The drawing under review shows one solid part. Ordinate dimensions are in mm from its lowest x, y, z. A direction names the side the tool comes from. Coordinates: 2 decimals unless noted, no trailing zeros. Write each loop counter-clockwise with the first axis right and the second up, starting at its lowest first coordinate (ties: lowest second). Pieces come first, ordered by that corner, then holes.
Q1. Add section B-B, the plane y = 18. Give the boundary of the cut face in (x, z), plus the area to 4 significant figures.
Q2. Clearance check with flat-ended pins moving along their axes: pin 1 Ø7 at (y, z) = (20, 115) entering from +X; pin 2 Ø13.5 at (y, z) = (20, 35) entering from +X; pin 3 Ø4 at (x, z) = (38, 134) entering from +Y. State where each tip first meets the part, or that it passes through.
Q3. Add section D-D, the plane z = 57.5. Give the boundary of the cut face in (x, y).
Q4. Machinability: for the marked faces 1 and 2, which of the approach directions +Z, -Z, +X, -X, +Y, -Y give a long, thin tool a straight path to every point of the face, cutting with its end or side? Answer none if there is none.
Q5. To check wall thickness, follow probe 1 along Z at (x, y) = (6.75, 20); probe 2 along Y at (x, z) = (7.75, 75); probe 3 along X at (y, z) = (5.25, 125). State the ranges of each line that lie inside material, in increasing order.
Q6. Add section C-C, the plane z = 113. Give the boundary of the cut face in (x, y), plus the area to 4 significant figures.
Q7. Add section A-A, the plane z = 75. Give the boundary of the cut face in (x, y).
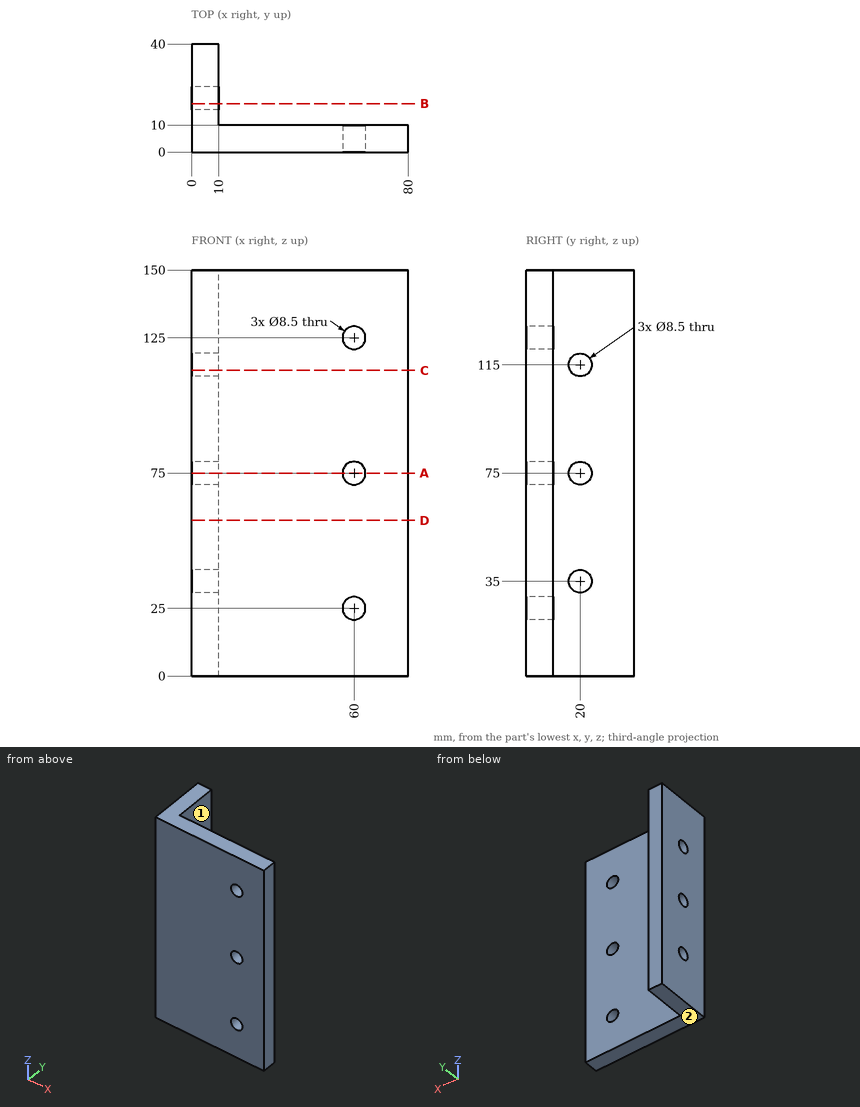
Here are the results:
1. outline: (0, 0) - (10, 0) - (10, 31.25) - (0, 31.25) - close; (0, 38.75) - (10, 38.75) - (10, 71.25) - (0, 71.25) - close; (0, 78.75) - (10, 78.75) - (10, 111.25) - (0, 111.25) - close; (0, 118.75) - (10, 118.75) - (10, 150) - (0, 150) - close
1. area: 1,275 mm2
2. pin 1: passes through
2. pin 2: stops at x = 10
2. pin 3: stops at y = 10
3. outline: (0, 0) - (80, 0) - (80, 10) - (10, 10) - (10, 40) - (0, 40) - close
4. face 1: +Z, -Z, +X, +Y
4. face 2: -Z, +X, -X, +Y, -Y
5. probe 1: z = 0 to 30.75, 39.25 to 70.75, 79.25 to 110.75, 119.25 to 150
5. probe 2: y = 0 to 15.75, 24.25 to 40
5. probe 3: x = 0 to 55.75, 64.25 to 80
6. outline: (0, 0) - (80, 0) - (80, 10) - (10, 10) - (10, 16.25) - (0, 16.25) - close; (0, 23.75) - (10, 23.75) - (10, 40) - (0, 40) - close
6. area: 1,025 mm2
7. outline: (0, 0) - (55.75, 0) - (55.75, 10) - (10, 10) - (10, 15.75) - (0, 15.75) - close; (0, 24.25) - (10, 24.25) - (10, 40) - (0, 40) - close; (64.25, 0) - (80, 0) - (80, 10) - (64.25, 10) - close
